from build123d import *

# Parameters (mm, degrees)
SKETCH1_W           = 184
SKETCH1_H           = 4
BOSS_EXTRUDE1_DEPTH = 74
CUT_EXTRUDE1_DEPTH  = 74


with BuildPart() as part:
    # Sketch1 → Boss-Extrude1 (new body)
    with BuildSketch(Plane.XY):
        with Locations((-92, 2)):
            Rectangle(SKETCH1_W, SKETCH1_H)
    extrude(amount=BOSS_EXTRUDE1_DEPTH)

    # Sketch2 → Cut-Extrude1 (cut)
    with BuildSketch(Plane(origin=(0, 4, 0), x_dir=(1, 0, 0), z_dir=(0, 1, 0))):
        Polygon((-70, -37), (-70, -29), (-86, -29), (-86, -45), (-70, -45), align=None)
    extrude(amount=-CUT_EXTRUDE1_DEPTH, mode=Mode.SUBTRACT)


solid = part.part
Input: part model. Units: mm. Frame: model coordinates. A direction names the side the tool comes from. Coordinates: 2 decimals unless noted, no trailing zeros. Order: outer loops, then holes, each group sorted by start corner. A loop starts at its lowest first (then second) coordinate and runs counter-clockwise, first axis right, second up. Notation, with made-up numbers: M 71,36.25 L 107,36.25 A31 ccw 107,71.25 Z; hole C -23.75,54.25 d8. An arc over 180 degrees is marked long. Answer as CSV lines item,"result".
1. Section A-A (z = 40). Return the cut outline in (x, y).
Reported:
outline,"M -184,0 L -86,0 L -86,4 L -184,4 Z; M -70,0 L 0,0 L 0,4 L -70,4 Z"
2. Access query for faces 4 (the flat face through (-93, 2, 0)), 5 (the flat face through (-86, 2, 37)). Directions: +Z, -Z, +X, -X, +Y, -Y. A direction counts if a zero-diameter tool reaches every point of the face in a straight line with its end or side. Return the directions, or none.
Reported:
face 4,"-Z, +X, -X, +Y, -Y"
face 5,"+Y, -Y"
3. Section B-B (y = 2). Return the cut outline in (x, z), then the cut area to 3 significant figures.
Reported:
outline,"M -184,0 L 0,0 L 0,74 L -184,74 Z; hole M -86,29 L -70,29 L -70,45 L -86,45 Z"
area,"13,400 mm2"
4. Pull-direction query (X, two-part tool) for faces 1 (the flat face through (-184, 2, 36)), 2 (the flat face through (-93, 4, 36)), 3 (the flat face through (-78, 2, 45)); classes: released by +X, released by -X, zero draft, split by the parting line, or undercut.
Reported:
face 1,"released by -X"
face 2,"zero draft"
face 3,"undercut"
5. Material intervals for line 1 (X direction, y = 1.3, z = 33.5), sorted ascending. Write a range as from..to.
Reported:
line 1,"-184..-86, -70..0"
